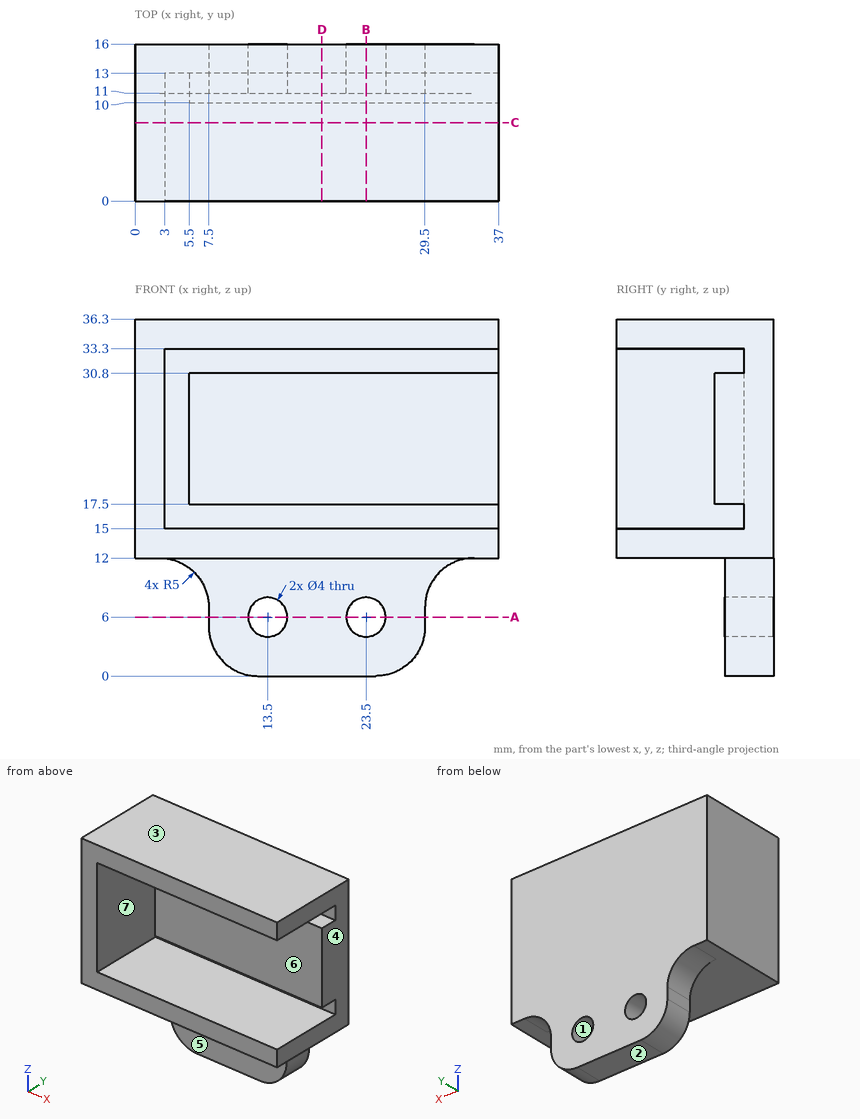
Can you work these out from the drawing? Everything is in mm from the part's minimum corner. A direction names the side the tool comes from. Round coordinates to 2 decimals unless told otherwise and drop trailing zeros. Loops run counter-clockwise (first coordinate to the right, second up) from the corner with the lowest first, then second, coordinate; pieces in that order, holes last. Notation, with made-up numbers: (0, -24) - (15, -24) arc R22 cw to (15, 6) - close; hole circle Ø4 at (-1.75, 50). An arc over 180 degrees is marked (long way). Write item = value, one per line. Start each with the question number.
(1) If we mould it in two halves opening along Z, with no side actions, what happens to the marked faces 1, 2 and 3? For each: released by +Z, released by -Z, zero draft, split by the parting line, or undercut.
(2) If we section it at A-A (z = 6): Please give me the cut outline in (x, y), and give its area (3 significant figures).
(3) If we section it at B-B (x = 23.5): Please give me the cut outline in (y, z).
(4) For P1, Ø9.5, axis at x = 18.5, z = 3.5, coming from the -Y side; P2, Ø2, axis at y = 14.5, z = 6, coming from the -X side; P3, Ø6.5, axis at x = 17.5, z = 25.5, coming from the -Y side, each with a flat end and sliding along its axis, tell me the tip position at first contact or that it passes through.
(5) If we section it at D-D (x = 19): Please give me the cut outline in (y, z), and give its area (3 significant figures).
(6) If I drill on probe 1 along X at (y, z) = (14.75, 6); probe 2 along Z at (x, y) = (23.5, 12.9); probe 3 along Z at (x, y) = (13.5, 13.7), over which ranges is the centre line in solid material (lowest first)? Write a range as [from, to].
(7) If we section it at C-C (y = 8): Please give me the cut outline in (x, z), and give its area (3 significant figures).
(8) For the marked faces 4, 5, 6 and 7, which set-ups out of +Z, -Z, +X, -X, +Y, -Y let a thin tool reach every point of the face, with its end or its side?
Ans:
q1.face_1 = undercut
q1.face_2 = released by -Z
q1.face_3 = released by +Z
q2.outline = (7.5, 11) - (11.5, 11) - (11.5, 16) - (7.5, 16) - close; (15.5, 11) - (21.5, 11) - (21.5, 16) - (15.5, 16) - close; (25.5, 11) - (29.5, 11) - (29.5, 16) - (25.5, 16) - close
q2.area = 70.0 mm²
q3.outline = (0, 12) - (11, 12) - (11, 8) - (16, 8) - (16, 36.3) - (0, 36.3) - (0, 33.3) - (13, 33.3) - (13, 30.8) - (10, 30.8) - (10, 17.5) - (13, 17.5) - (13, 15) - (0, 15) - close; (11, 0) - (16, 0) - (16, 4) - (11, 4) - close
q4.P1 = 11
q4.P2 = 7.5
q4.P3 = 10
q5.outline = (0, 12) - (11, 12) - (11, 0) - (16, 0) - (16, 36.3) - (0, 36.3) - (0, 33.3) - (13, 33.3) - (13, 30.8) - (10, 30.8) - (10, 17.5) - (13, 17.5) - (13, 15) - (0, 15) - close
q5.area = 251 mm²
q6.probe_1 = [7.5, 11.5], [15.5, 21.5], [25.5, 29.5]
q6.probe_2 = [0, 4], [8, 15], [17.5, 30.8], [33.3, 36.3]
q6.probe_3 = [0, 4], [8, 36.3]
q7.outline = (0, 12) - (37, 12) - (37, 15) - (3, 15) - (3, 33.3) - (37, 33.3) - (37, 36.3) - (0, 36.3) - close
q7.area = 277 mm²
q8.face_4 = +Z, -Z, +X, +Y, -Y
q8.face_5 = -Z, +X, -X, -Y
q8.face_6 = +X, -Y
q8.face_7 = -Y
